```python
from build123d import *

# Parameters (mm, degrees)
SKETCH_3_R          = 9.5
EXTRUDE_1_DEPTH     = 1
EXTRUDE_START       = -1
EXTRUDE_2_DEPTH     = 1
FILLET_2_R          = 13
SKETCH_5_R          = 1.15
CUT_EXTRUDE_1_DEPTH = 58.922235489
SKETCH_6_R          = 9.5
CUT_EXTRUDE_2_DEPTH = 58.922235489
FILLET_3_R          = 8
FILLET_4_R          = 7
SKETCH_7_R          = 1.08334678
CUT_EXTRUDE_4_DEPTH = 10
CUT_EXTRUDE_5_DEPTH = 10


with BuildPart() as part:
    # 草图3 → 凸台-拉伸1 (new body)
    with BuildSketch(Plane.XY):
        with BuildLine():
            Line((-11, 0), (-11, -33))
            Line((-11, -33), (35.74, -33))
            ThreePointArc((35.74, -33), (46.48709263, -19.65479212), (31.157424305, -12))
            Line((31.157424305, -12), (9, -12))
            Line((9, -12), (9, -6.32455532))
            ThreePointArc((9, -6.32455532), (3.31662479, 10.488088482), (-11, 0))
        make_face()
        Circle(SKETCH_3_R, mode=Mode.SUBTRACT)
        with Locations((35.74, -22)):
            Circle(SKETCH_3_R, mode=Mode.SUBTRACT)
    extrude(amount=EXTRUDE_1_DEPTH)

    # 草图4 → 凸台-拉伸2 (add)
    with BuildSketch(Plane.XY.offset(1).offset(EXTRUDE_START)):
        with BuildLine():
            Line((35.74, -33), (-12.210859555, -34.674480913))
            Line((-12.210859555, -34.674480913), (-11, 0))
            ThreePointArc((-11, 0), (3.31662479, 10.488088482), (9, -6.32455532))
            Line((9, -6.32455532), (9, -12))
            Line((9, -12), (31.157424305, -12))
            ThreePointArc((31.157424305, -12), (46.48709263, -19.65479212), (35.74, -33))
        make_face()
    extrude(amount=EXTRUDE_2_DEPTH)

    # 圆角2
    fillet_2_edges = [part.edges().sort_by_distance(p)[0] for p in [
        (-12.210859555, -34.674480913, 0.5),
    ]]
    fillet(fillet_2_edges, radius=FILLET_2_R)

    # 草图5 → 切除-拉伸1 (cut, through all)
    with BuildSketch(Plane.XY.offset(1)):
        with Locations((-8, -22.5)):
            Circle(SKETCH_5_R)
        with Locations((8, -22.5)):
            Circle(SKETCH_5_R)
    extrude(amount=-CUT_EXTRUDE_1_DEPTH, mode=Mode.SUBTRACT)

    # 草图6 → 切除-拉伸2 (cut, through all)
    with BuildSketch(Plane.XY.offset(1)):
        Circle(SKETCH_6_R)
        with Locations((35.642814002, -22)):
            Circle(SKETCH_6_R)
    extrude(amount=-CUT_EXTRUDE_2_DEPTH, mode=Mode.SUBTRACT)

    # 圆角3
    # the kernel refuses this fillet: 8 mm, written as the material it adds along each edge
    with BuildSketch(Plane(origin=(9, -12, 0), x_dir=(0, 1, 0), z_dir=(0, 0, 1))) as fillet_3_piece_1:
        with BuildLine():
            CenterArc((8, -7.654831322), FILLET_3_R, 106.89204914, 73.10795086)
            Line((0, -7.654831322), (-0.16, -7.654831322))
            Line((-0.16, -7.654831322), (-0.16, 0))
            Line((-0.16, 0), (0, 0.16))
            ThreePointArc((0, 0.16), (2.83772234, 0.16), (5.628953573, 0.153096626))
            Line((5.628953573, 0.153096626), (5.67544468, 0))
        make_face()
    extrude(amount=1)

    # 圆角4
    fillet_4_edges = [part.edges().sort_by_distance(p)[0] for p in [
        (9, -6.32455532, 0.5),
    ]]
    fillet(fillet_4_edges, radius=FILLET_4_R)

    # 草图7 → 切除-拉伸4 (cut)
    with BuildSketch(Plane.XY.offset(1)):
        with Locations((13.142814002, -14)):
            Circle(SKETCH_7_R)
        with Locations((13.142814002, -30)):
            Circle(SKETCH_7_R)
    extrude(amount=-CUT_EXTRUDE_4_DEPTH, mode=Mode.SUBTRACT)

    # 草图8 → 切除-拉伸5 (cut)
    with BuildSketch(Plane.XY.offset(1)):
        with BuildLine():
            Line((16.157202734, -30.291096898), (16.157202734, -13.355657228))
            Line((16.157202734, -13.355657228), (23.81874567, -13.355657228))
            ThreePointArc((23.81874567, -13.355657228), (25.535376674, -14.32941262), (25.580428982, -16.302479233))
            ThreePointArc((25.580428982, -16.302479233), (24.200275644, -21.822246327), (25.614952461, -27.333266333))
            ThreePointArc((25.614952461, -27.333266333), (25.579064672, -29.3119639), (23.859230214, -30.291096898))
            Line((23.859230214, -30.291096898), (16.157202734, -30.291096898))
        make_face()
        with BuildLine():
            Line((-1.844212644, -26.7628803), (8.691309214, -26.7628803))
            ThreePointArc((8.691309214, -26.7628803), (9.751969386, -27.202220128), (10.191309214, -28.2628803))
            Line((10.191309214, -28.2628803), (10.191309214, -30.26653293))
            ThreePointArc((10.191309214, -30.26653293), (9.751969386, -31.327193102), (8.691309214, -31.76653293))
            Line((8.691309214, -31.76653293), (-1.844212644, -31.76653293))
            ThreePointArc((-1.844212644, -31.76653293), (-2.904872816, -31.327193102), (-3.344212644, -30.26653293))
            Line((-3.344212644, -30.26653293), (-3.344212644, -28.2628803))
            ThreePointArc((-3.344212644, -28.2628803), (-2.904872816, -27.202220128), (-1.844212644, -26.7628803))
        make_face()
        with BuildLine():
            Line((-8.796911022, -16.052867786), (-8.796911022, -12.380312846))
            ThreePointArc((-8.796911022, -12.380312846), (-7.815486406, -10.659120182), (-5.834406834, -10.627148368))
            ThreePointArc((-5.834406834, -10.627148368), (0.968228408, -12.084664633), (7.452020697, -9.562634212))
            ThreePointArc((7.452020697, -9.562634212), (7.978826228, -9.507761331), (8.259361329, -9.957022011))
            Line((8.259361329, -9.957022011), (8.259361329, -10.859557769))
            ThreePointArc((8.259361329, -10.859557769), (7.914413338, -11.982412545), (6.99855848, -12.717940822))
            Line((6.99855848, -12.717940822), (-6.057713871, -17.911250839))
            ThreePointArc((-6.057713871, -17.911250839), (-7.919765799, -17.707919794), (-8.796911022, -16.052867786))
        make_face()
    extrude(amount=-CUT_EXTRUDE_5_DEPTH, mode=Mode.SUBTRACT)


solid = part.part
```
The model under review builds one solid part; all positions refer to its coordinate system, in mm. Round coordinates to 2 decimals unless told otherwise and drop trailing zeros. Loops run counter-clockwise (first coordinate to the right, second up) from the corner with the lowest first, then second, coordinate; pieces in that order, holes last. Notation, with made-up numbers: M 62.5,21.5 L 87.5,21.5 A27 cw 87.5,42.5 Z; hole C 79.5,-19 d1. An arc over 180 degrees is marked long. Put each result on its own line as item: value.
Q1. For pin 1 (0.5 mm diameter, centred on y = -29.5, z = 0.5, fed in from +X); pin 2 (0.5 mm diameter, centred on y = -10.5, z = 0.5, fed in from -X), all flat-tipped, find the tip position at first contact; note any pin that passes through.
Result set:
pin 1: stops at x = 44.01
pin 2: stops at x = -11.38
Q2. Consider section B-B, the plane x = 19.5. Give the boundary of the cut face in (y, z).
Result set:
outline: M -33.57,0 L -30.29,0 L -30.29,1 L -33.57,1 Z; M -13.36,0 L -12,0 L -12,1 L -13.36,1 Z
Q3. Mouldability with a two-part tool opening along Y and no side actions: class faces 1 (the cylindrical face through (-7.9, -17.72, 0.51)), 2 (the flat face through (11, -18, 0)), 3 (the cylindrical face through (46.54, -19.92, 0.49)) as released by +Y, released by -Y, zero draft, split by the parting line, or undercut.
Result set:
face 1: undercut
face 2: zero draft
face 3: split by the parting line
Q4. Consider section D-D, the plane x = 0. Give the boundary of the cut face in (y, z).
Result set:
outline: M -34.13,0 L -31.77,0 L -31.77,1 L -34.13,1 Z; M -26.76,0 L -15.5,0 L -15.5,1 L -26.76,1 Z; M -12.12,0 L -9.5,0 L -9.5,1 L -12.12,1 Z; M 9.5,0 L 11,0 L 11,1 L 9.5,1 Z
Q5. To check wall thickness, follow L1, parallel to X at y = -24, z = 0.35; L2, parallel to Y at x = 14, z = 0.55; L3, parallel to Y at x = 36, z = 0.45. State the ranges of each line that lie inside material, in increasing order.
Result set:
L1: x = -11.43 to 16.16, 24.41 to 26.36, 44.93 to 46.56
L2: y = -33.76 to -30.66, -29.34 to -14.66, -13.34 to -11.18
L3: y = -33 to -31.49, -12.51 to -11
Q6. Consider section A-A, the plane y = 2.5. Give the boundary of the cut face in (x, z), then the cut area to 3 significant figures.
Result set:
outline: M -10.71,0 L -9.17,0 L -9.17,1 L -10.71,1 Z; M 9.17,0 L 10.71,0 L 10.71,1 L 9.17,1 Z
area: 3.09 mm²
Q7. Consider section C-C, the plane y = -24.5. Give the boundary of the cut face in (x, z).
Result set:
outline: M -11.31,0 L 16.16,0 L 16.16,1 L -11.31,1 Z; M 24.52,0 L 26.48,0 L 26.48,1 L 24.52,1 Z; M 44.81,0 L 46.45,0 L 46.45,1 L 44.81,1 Z
